Solid Edge part; units mm, degrees
sketch "Sketch1" plane through (0, 0, 0) normal (0, 0, 1) x (1, 0, 0)
  line L0 (-105, -65) -> (105, -65)
  line L1 (105, -65) -> (105, 65)
  line L2 (105, 65) -> (-105, 65)
  line L3 (-105, 65) -> (-105, -65)
extrude "Protrusion1" add sketch "Sketch1" against normal blind 30
sketch "Sketch2" plane through (0, 0, 0) normal (0, 0, 1) x (0, 1, 0)
  circle A0 centre (0, 35) radius 51.25
extrude "Recorte_Extrudado_4" cut sketch "Sketch2" against normal blind 30
sketch "Sketch3" plane through (0, 0, 0) normal (0, 0, 1) x (0, 1, 0)
  circle A0 centre (0, 35) radius 53.7
extrude "Recorte_Extrudado_5" cut sketch "Sketch3" against normal blind 23
sketch "Sketch4" plane through (0, 0, 0) normal (0, 0, 1) x (0, 1, 0)
  circle A0 centre (0, 35) radius 57.95
extrude "Recorte_Extrudado_6" cut sketch "Sketch4" against normal blind 16
Geometry: final body of the model. Coordinates: model frame, mm. A direction names the side the tool comes from. Coordinates: 2 decimals unless noted, no trailing zeros. Order: outer loops, then holes, each group sorted by start corner. A loop starts at its lowest first (then second) coordinate and runs counter-clockwise, first axis right, second up.
(1) Section query C-C (x = -35). Return the cut outline in (y, z).
(2) Section query B-B (z = -5.5). Return the cut outline in (x, y).
(3) Material intervals for probe 1 along Y at (x, z) = (-35, -19.5); probe 2 along Y at (x, z) = (-35, -8.5); probe 3 along X at (y, z) = (0, -27), sorted ascending.
(4) Section query A-A (y = 0). Return the cut outline in (x, z), plus the area to 3 significant figures.
(5) Access query for faces 1 (the face through (-18.1, -51.2, -16)), 2 (the face through (-105, 1, -15)). Directions: +Z, -Z, +X, -X, +Y, -Y. A direction counts if a zero-diameter tool reaches every point of the face in a straight line with its end or side. Return the directions, or none.
(6) Section query D-D (z = -18.5). Return the cut outline in (x, y), plus the area to 3 significant figures.
(7) Draft query along Y for faces 3 (the face through (-7, -44, -23)), 4 (the face through (22, 1, -30)), 5 (the face through (1, 65, -15)). Return one class per face: pulls with the +Y half, pulls with the -Y half, needs draft (parallel to the pull), parting line crosses it, or undercut.
Solution:
1. outline: (-65, -30) - (-51.25, -30) - (-51.25, -23) - (-53.7, -23) - (-53.7, -16) - (-57.95, -16) - (-57.95, 0) - (-65, 0) - close; (51.25, -30) - (65, -30) - (65, 0) - (57.95, 0) - (57.95, -16) - (53.7, -16) - (53.7, -23) - (51.25, -23) - close
2. outline: (-105, -65) - (105, -65) - (105, 65) - (-105, 65) - close; hole circle Ø115.9 at (-35, 0)
3. probe 1: y = -65 to -53.7, 53.7 to 65
3. probe 2: y = -65 to -57.95, 57.95 to 65
3. probe 3: x = -105 to -86.25, 16.25 to 105
4. outline: (-105, -30) - (-86.25, -30) - (-86.25, -23) - (-88.7, -23) - (-88.7, -16) - (-92.95, -16) - (-92.95, 0) - (-105, 0) - close; (16.25, -30) - (105, -30) - (105, 0) - (22.95, 0) - (22.95, -16) - (18.7, -16) - (18.7, -23) - (16.25, -23) - close
4. area: 2,980 mm2
5. face 1: +Z
5. face 2: +Z, -Z, -X, +Y, -Y
6. outline: (-105, -65) - (105, -65) - (105, 65) - (-105, 65) - close; hole circle Ø107.4 at (-35, 0)
6. area: 18,200 mm2
7. face 3: undercut
7. face 4: needs draft
7. face 5: pulls with the +Y half
